Answer from the drawing. Dimensions are ordinates in mm from the lowest x, y and z of the part. A direction names the side the tool comes from. Round coordinates to 2 decimals unless told otherwise and drop trailing zeros. Loops run counter-clockwise (first coordinate to the right, second up) from the corner with the lowest first, then second, coordinate; pieces in that order, holes last. Notation, with made-up numbers: M -2.75,-26.75 L 55.25,-26.75 A11 ccw 55.25,-9.75 Z; hole C 22,41 d7. An arc over 180 degrees is marked long. Answer as a JSON object with one key per item and string values.
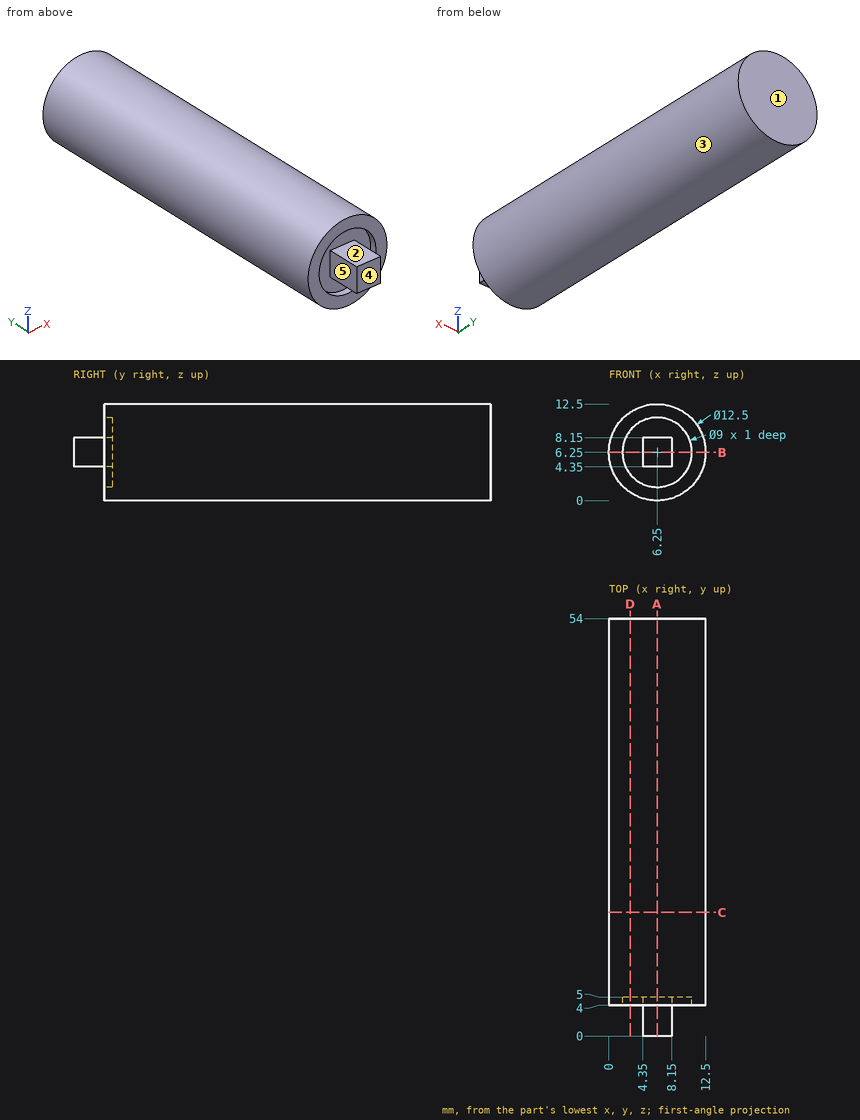
Item 1: Determine the mould class of the marked faces 1, 2 and 3 for opening direction X: released by +X, released by -X, zero draft, split by the parting line, or undercut.
Values follow:
{"face 1": "zero draft", "face 2": "undercut", "face 3": "split by the parting line"}
Item 2: The part is cut by section C-C (y = 16). Give the vertices of the cut face in (x, z).
Values follow:
{"outline": "C 6.25,6.25 d12.5"}
Item 3: Flat-ended cylindrical pins translate along their axes: P1, Ø1, axis at x = 8, y = 44.5, coming from the -Z side; P2, Ø1.9, axis at x = 6.5, y = 2, coming from the +Z side; P3, Ø1.5, axis at x = 4.5, z = 10, coming from the -Y side. Find the tip coordinate at first contact, or state that the pin passes through.
Values follow:
{"P1": "z = 0.13", "P2": "z = 8.15", "P3": "y = 4"}
Item 4: The part is cut by section A-A (x = 6.25). Give the vertices of the cut face in (y, z).
Values follow:
{"outline": "M 0,4.35 L 5,4.35 L 5,1.75 L 4,1.75 L 4,0 L 54,0 L 54,12.5 L 4,12.5 L 4,10.75 L 5,10.75 L 5,8.15 L 0,8.15 Z"}
Item 5: Which of the six approach directions +Z, -Z, +X, -X, +Y, -Y give full straight-line access (tool end or side, diameter ignored) to the marked faces 4 and 5?
Values follow:
{"face 4": "+Z, -Z, +X, -X, -Y", "face 5": "-Y"}
Item 6: Straight lines are drawn through the part: line 1 (Z direction, x = 6.25, y = 4.5); line 2 (Y direction, x = 11, z = 5.75); line 3 (Y direction, x = 9.25, z = 5). For each, find the intervals that lie inside material, in ascending order.
Values follow:
{"line 1": "0 to 1.75, 4.35 to 8.15, 10.75 to 12.5", "line 2": "4 to 54", "line 3": "5 to 54"}
Item 7: The part is cut by section D-D (x = 2.75). Give the vertices of the cut face in (y, z).
Values follow:
{"outline": "M 4,1.07 L 54,1.07 L 54,11.43 L 4,11.43 L 4,9.08 L 5,9.08 L 5,3.42 L 4,3.42 Z"}
Item 8: The part is cut by section B-B (z = 6.25). Give the vertices of the cut face in (x, y).
Values follow:
{"outline": "M 0,4 L 1.75,4 L 1.75,5 L 4.35,5 L 4.35,0 L 8.15,0 L 8.15,5 L 10.75,5 L 10.75,4 L 12.5,4 L 12.5,54 L 0,54 Z"}
